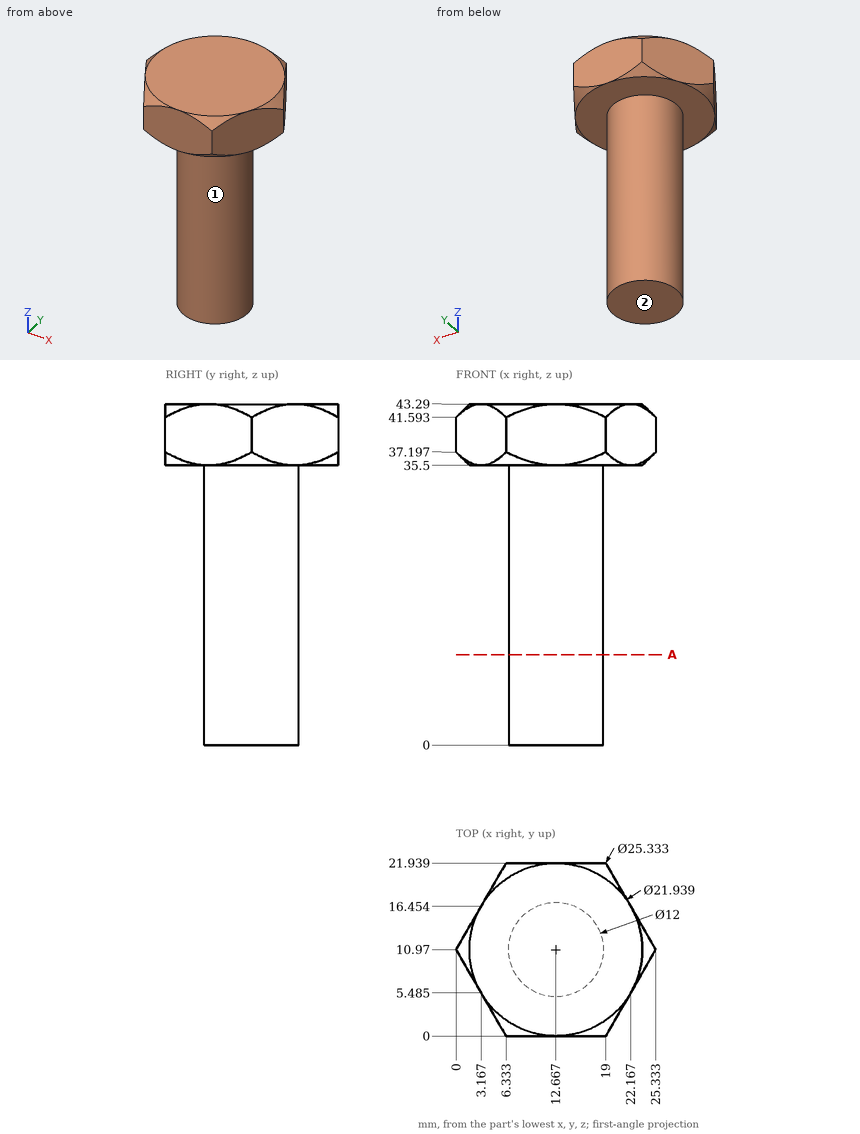
Geometry check sheet. Reference: drawing and pictorial views, mm from the part's lowest x, y, z. A direction names the side the tool comes from. Give positions to 0.01 mm unless a question says otherwise; leave off trailing zeros. Order: outer loops, then holes, each group sorted by start corner. A loop starts at its lowest first (then second) coordinate and runs counter-clockwise, first axis right, second up. Notation, with made-up numbers: M 29,78 L 69,78 A21 cw 69,106 Z; hole C 40,58.25 d7. An arc over 180 degrees is marked long. Answer in a Markdown table with one row per item. Add a question column.
Item 1: Section check A-A, the plane z = 11.5. Enter the section's corners in (x, y).
Item 2: Gauge pin test, flat ends, axial feed: pin 1 (3 mm diameter, centred on y = 11, z = 16, fed in from -X); pin 2 (10 mm diameter, centred on y = 4.5, z = 19, fed in from -X); pin 3 (4 mm diameter, centred on y = 12.5, z = 7.5, fed in from +X). Record the tip position at first contact, or that the pin passes through.
Item 3: Scan lines: probe 1 along Y at (x, z) = (13, 2); probe 2 along Z at (x, y) = (5.25, 15); probe 3 along X at (y, z) = (20.75, 38.5) (1 decimal). Record each from-to range of solid material in increasing order. Write a range as from..to.
Item 4: Tool access check on the marked faces 1 and 2. Record the directions out of +Z, -Z, +X, -X, +Y, -Y that give a thin tool (end or side, any length) a straight path to the whole face; none if there is none.
Filled sheet:
| question | item | result |
|---|---|---|
| 1 | outline | C 12.67,10.97 d12 |
| 2 | pin 1 | stops at x = 6.67 |
| 2 | pin 2 | stops at x = 6.85 |
| 2 | pin 3 | stops at x = 18.67 |
| 3 | probe 1 | y = 4.98..16.96 |
| 3 | probe 2 | z = 35.5..43.29 |
| 3 | probe 3 | x = 5.6..19.7 |
| 4 | face 1 | -Z |
| 4 | face 2 | -Z, +X, -X, +Y, -Y |
